from build123d import *

# Parameters (mm, degrees)
F0_W     = 80
F0_H     = 80
F0_R     = 2.5423391552
F1_DEPTH = 12.5
F2_R     = 5


with BuildPart() as f1:
    # F0 (on Front) → F1 (new body, symmetric)
    with BuildSketch(Plane.XZ):
        Rectangle(F0_W, F0_H)
        with Locations((-34.4576608448, -34.4576608448)):
            Circle(F0_R, mode=Mode.SUBTRACT)
        with BuildLine():
            Line((-37.9351268711, -2.219493022), (-14.3494285056, 10.01718032))
            ThreePointArc((-14.3494285056, 10.01718032), (-17.4625571186, 1.1441585906), (-15.5338058985, -8.0592105263))
            Line((-15.5338058985, -8.0592105263), (0, -38))
            ThreePointArc((0, -38), (-26.0735427701, -27.6436315888), (-37.9351268711, -2.219493022))
        make_face(mode=Mode.SUBTRACT)
        with Locations((34.4576608448, -34.4576608448)):
            Circle(F0_R, mode=Mode.SUBTRACT)
        with BuildLine():
            Line((8.0592105263, -15.5338058985), (38, 0))
            ThreePointArc((38, 0), (27.6436315888, -26.0735427701), (2.219493022, -37.9351268711))
            Line((2.219493022, -37.9351268711), (-10.01718032, -14.3494285056))
            ThreePointArc((-10.01718032, -14.3494285056), (-1.1441585906, -17.4625571186), (8.0592105263, -15.5338058985))
        make_face(mode=Mode.SUBTRACT)
        with BuildLine():
            Line((-8.0592105263, 15.5338058985), (-38, 0))
            ThreePointArc((-38, 0), (-27.6436315888, 26.0735427701), (-2.219493022, 37.9351268711))
            Line((-2.219493022, 37.9351268711), (10.01718032, 14.3494285056))
            ThreePointArc((10.01718032, 14.3494285056), (1.1441585906, 17.4625571186), (-8.0592105263, 15.5338058985))
        make_face(mode=Mode.SUBTRACT)
        with Locations((-34.4576608448, 34.4576608448)):
            Circle(F0_R, mode=Mode.SUBTRACT)
        with BuildLine():
            Line((15.5338058985, 8.0592105263), (0, 38))
            ThreePointArc((0, 38), (26.0735427701, 27.6436315888), (37.9351268711, 2.219493022))
            Line((37.9351268711, 2.219493022), (14.3494285056, -10.01718032))
            ThreePointArc((14.3494285056, -10.01718032), (17.4625571186, -1.1441585906), (15.5338058985, 8.0592105263))
        make_face(mode=Mode.SUBTRACT)
        with Locations((34.4576608448, 34.4576608448)):
            Circle(F0_R, mode=Mode.SUBTRACT)
    extrude(amount=F1_DEPTH, both=True)

    # F2
    f2_edges = [f1.edges().sort_by_distance(p)[0] for p in [
        (10.01718, 0, 14.349429),
        (-14.349429, 0, 10.01718),
        (-10.01718, 0, -14.349429),
        (14.349429, 0, -10.01718),
    ]]
    fillet(f2_edges, radius=F2_R)


solid = f1.part
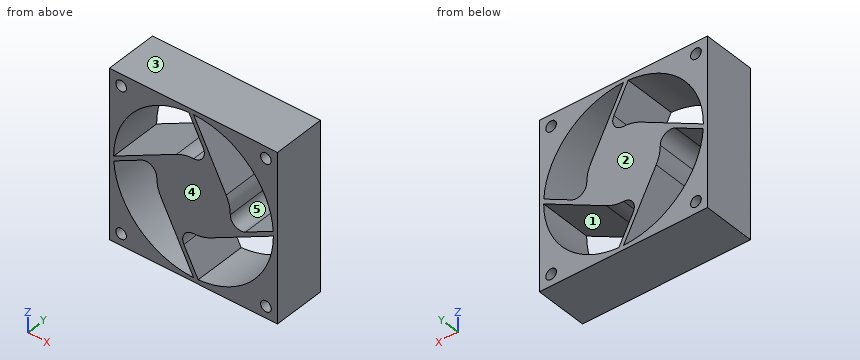
The listing builds one solid part. Answer for the finished solid, in the listing's coordinates (mm). Face numbers are marked on the shaded views. A direction names the side the tool comes from. Coordinates: 2 decimals unless noted, no trailing zeros. Write each loop counter-clockwise with the first axis right and the second up, starting at its lowest first coordinate (ties: lowest second). Pieces come first, ordered by that corner, then holes. Notation, with made-up numbers: M -13.75,1 L -5.75,1 A18 cw -5.75,33 Z; hole C -14,-29.5 d6. An arc over 180 degrees is marked long. Write each question's results on one line, items separated by ' | '.
Item 1: The part is cut by section B-B on z = 12. Determine the outline of the cut face in (x, y).
Answer below:
outline: M -40,-12.5 L -36.06,-12.5 L -36.06,12.5 L -40,12.5 Z; M -14.87,-12.5 L 13.49,-12.5 L 13.49,12.5 L -14.87,12.5 Z; M 36.06,-12.5 L 40,-12.5 L 40,12.5 L 36.06,12.5 Z
Item 2: For a pull along Z with two mould halves and no side action, classify the marked faces 1, 2 and 3 as released by +Z, released by -Z, zero draft, split by the parting line, or undercut.
Answer below:
face 1: undercut | face 2: zero draft | face 3: released by +Z
Item 3: The part is cut by section C-C on y = 4.5. State how many separate pieces and enclosed holes the cut face has, and give its area (3 significant figures).
Answer below:
separate pieces: 1 | enclosed holes: 8 | area: 3,070 mm2
Item 4: The part is cut by section A-A on x = 20. Determine the outline of the cut face in (y, z).
Answer below:
outline: M -12.5,-40 L 12.5,-40 L 12.5,-32.31 L -12.5,-32.31 Z; M -12.5,-9.34 L 12.5,-9.34 L 12.5,-4.49 L -12.5,-4.49 Z; M -12.5,32.31 L 12.5,32.31 L 12.5,40 L -12.5,40 Z
Item 5: Given P1, Ø3, axis at x = 34.46, z = 34.46, coming from the -Y side, flat-ended and moving along its own axis, determine where the tip first touches the part or whether it passes through.
Answer below:
P1: through
Item 6: Which of the six approach directions +Z, -Z, +X, -X, +Y, -Y give full straight-line access (tool end or side, diameter ignored) to the marked faces 4 and 5?
Answer below:
face 4: +Z, -Z, +X, -X, -Y | face 5: +Y, -Y
Item 7: Consider probe 1 along Z at (x, y) = (2.5, -3.75); probe 2 along Z at (x, y) = (-8.5, -8.25); probe 3 along Z at (x, y) = (4, 10.25). Determine where each line is inside the solid, lowest interval first. Write a range as [from, to].
Answer below:
probe 1: [-40, -37.92], [-17.32, 18.08], [28.84, 33.18], [37.92, 40] | probe 2: [-40, -37.04], [-21.62, 15.31], [37.04, 40] | probe 3: [-40, -37.79], [-17.04, 19.3], [25.95, 30.29], [37.79, 40]
